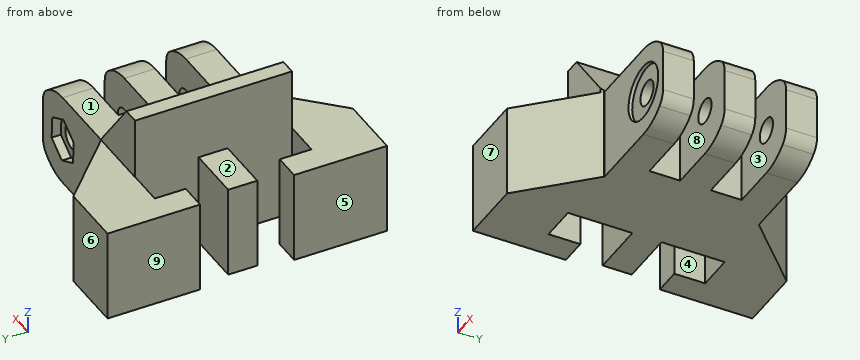
```python
from build123d import *

# Parameters (mm, degrees)
BOSS_EXTRUDE1_DEPTH = 15
FILLET1_R           = 7.5
SKETCH2_R           = 2
CUT_EXTRUDE1_DEPTH  = 56.055379886
SKETCH3_R           = 4.5
CUT_EXTRUDE2_DEPTH  = 0.6
CUT_EXTRUDE3_DEPTH  = 1.5
SKETCH5_W           = 11.340962939
SKETCH5_H           = 24.83561836
CUT_EXTRUDE4_DEPTH  = 56.308893581
FILLET2_R           = 3
SKETCH6_W           = 2.415249458
SKETCH6_H           = 25.484257417
BOSS_EXTRUDE2_DEPTH = 10
CHAMFER1_SIZE       = 8
CHAMFER1_SIZE_2     = 10.239533058


# Some blends are built 0.0001 mm under size
with BuildPart() as part:
    # Sketch1 → Boss-Extrude1 (new body)
    with BuildSketch(Plane.XY):
        Polygon((27.272753899, 35.386642786), (20.490738927, 35.386642786), (20.490738927, 35.487239574), (10.340798609, 45.376041655), (0, 45.376041655), (0, 30.338888881), (4.365624999, 30.338888881), (4.365624999, 35.365972213), (10.274652775, 35.365972213), (10.274652775, 25.091319438), (1.278819444, 25.091319438), (1.278819444, 20.372916662), (10.274652775, 20.372916662), (10.274652775, 9.921874998), (4.365624999, 9.921874998), (4.365624999, 15.081249996), (0, 15.081249996), (0, 0), (10.340798609, 0), (20.490738927, 10.304280596), (20.490738927, 10.386962888), (27.272753899, 10.386962888), (39.772593849, 10.386962888), (39.772593849, 15.38338487), (24.772648106, 15.38338487), (24.772648106, 20.383251948), (39.772593849, 20.383251948), (39.772593849, 22.886802837), (39.772593849, 25.362792962), (24.772648106, 25.362792962), (24.772648106, 30.36266004), (39.772593849, 30.36266004), (39.772593849, 35.386642786), align=None)
    extrude(amount=BOSS_EXTRUDE1_DEPTH)

    # Fillet1
    fillet1_edges = [part.edges().sort_by_distance(p)[0] for p in [
        (39.772593849, 32.874651413, 0),
        (39.772593849, 22.873022455, 0),
        (39.772593849, 12.885173879, 0),
        (39.772593849, 32.874651413, 15),
        (39.772593849, 22.873022455, 15),
        (39.772593849, 12.885173879, 15),
    ]]
    fillet(fillet1_edges, radius=FILLET1_R - 0.0001)  # a hair under: the kernel refuses the full size

    # Sketch2 → Cut-Extrude1 (cut, through all)
    with BuildSketch(Plane.XZ.offset(-10.386962888)):
        with Locations(Location((32.272593849, 7.5, 0), (0, 0, 270))):
            Circle(SKETCH2_R)
    extrude(amount=-CUT_EXTRUDE1_DEPTH, mode=Mode.SUBTRACT)

    # Sketch3 → Cut-Extrude2 (cut)
    with BuildSketch(Plane(origin=(0, 10.386962888, 0), x_dir=(-1, 0, 0), z_dir=(0, -1, 0))):
        with Locations(Location((-32.272593849, -7.5, 0), (0, 0, 90))):
            Circle(SKETCH3_R)
    extrude(amount=-CUT_EXTRUDE2_DEPTH, mode=Mode.SUBTRACT)

    # Sketch4 → Cut-Extrude3 (cut)
    with BuildSketch(Plane(origin=(0, 35.386642786, 0), x_dir=(1, 0, 0), z_dir=(0, 1, 0))):
        Polygon((35.624325063, -5.818215869), (32.491991675, -3.756423556), (29.14026046, -5.438207687), (28.920862634, -9.181784131), (32.053196023, -11.243576444), (35.404927237, -9.561792313), align=None)
    extrude(amount=-CUT_EXTRUDE3_DEPTH, mode=Mode.SUBTRACT)

    # Sketch5 → Cut-Extrude4 (cut, through all)
    with BuildSketch(Plane(origin=(0, 35.386642786, 0), x_dir=(1, 0, 0), z_dir=(0, 1, 0))):
        with Locations((43.904057381, -8.645001066)):
            Rectangle(SKETCH5_W, SKETCH5_H)
    extrude(amount=-CUT_EXTRUDE4_DEPTH, mode=Mode.SUBTRACT)

    # Fillet2
    fillet2_edges = [part.edges().sort_by_distance(p)[0] for p in [
        (38.233575911, 12.885173879, 2.948374426),
        (38.233575911, 12.885173879, 12.051625574),
        (38.233575911, 22.873022455, 12.051625574),
        (38.233575911, 22.873022455, 2.948374426),
        (38.233575911, 32.874651413, 12.051625574),
        (38.233575911, 32.874651413, 2.948374426),
    ]]
    fillet(fillet2_edges, radius=FILLET2_R)

    # Sketch6 → Boss-Extrude2 (add)
    with BuildSketch(Plane.XY.offset(15)):
        with Locations((11.482277504, 22.664003707)):
            Rectangle(SKETCH6_W, SKETCH6_H)
    extrude(amount=BOSS_EXTRUDE2_DEPTH)

    # Chamfer1
    # the kernel refuses this chamfer: 10.239533058, 8 mm, written as the material it adds along each edge
    with BuildSketch(Plane(origin=(12.689902233, 9.921874998, 15), x_dir=(0.9992360216896828, 0, -0.03908161918057676), z_dir=(0, 1, 0))) as chamfer1_piece_1_section:
        Polygon((CHAMFER1_SIZE * 0.99923602169, -CHAMFER1_SIZE * 0.0390816191806), (-CHAMFER1_SIZE_2 * 0.0390816191788, -CHAMFER1_SIZE_2 * 0.999236021645), (0, 0), align=None)
    chamfer1_piece_1 = extrude(amount=25.484257417, mode=Mode.PRIVATE)
    chamfer1_piece_1 = split(chamfer1_piece_1, bisect_by=Plane(origin=(20.793346788, 10.386962888, 14.678631533), z_dir=(0, 1, 0)), keep=Keep.TOP, mode=Mode.PRIVATE)
    chamfer1_piece_1 = split(chamfer1_piece_1, bisect_by=Plane(origin=(20.737221422, 10.554511111, 14.678631533), z_dir=(0.7124220763083485, -0.7017512274221556, 0)), keep=Keep.TOP, mode=Mode.PRIVATE)
    add(chamfer1_piece_1)
    with BuildSketch(Plane(origin=(12.689902233, 9.921874998, 15), x_dir=(0.9992360216896828, 0, -0.03908161918057676), z_dir=(0, 1, 0))) as chamfer1_piece_2_section:
        Polygon((CHAMFER1_SIZE * 0.99923602169, -CHAMFER1_SIZE * 0.0390816191806), (-CHAMFER1_SIZE_2 * 0.0390816191788, -CHAMFER1_SIZE_2 * 0.999236021645), (0, 0), align=None)
    chamfer1_piece_2 = extrude(amount=25.484257417, mode=Mode.PRIVATE)
    chamfer1_piece_2 = split(chamfer1_piece_2, bisect_by=Plane(origin=(15.274873459, 10.386962888, 18.392715242), z_dir=(0, -1, 0)), keep=Keep.TOP, mode=Mode.PRIVATE)
    chamfer1_piece_2 = split(chamfer1_piece_2, bisect_by=Plane(origin=(20.490738927, 10.154752313, 18.392715242), z_dir=(-1, 0, 0)), keep=Keep.TOP, mode=Mode.PRIVATE)
    chamfer1_piece_2 = split(chamfer1_piece_2, bisect_by=Plane(origin=(17.84740539, 7.620752455, 18.392715242), z_dir=(-0.7124220763083485, 0.7017512274221556, 0)), keep=Keep.TOP, mode=Mode.PRIVATE)
    chamfer1_piece_2 = split(chamfer1_piece_2, bisect_by=Plane(origin=(15.274873459, 10.154752313, 25), z_dir=(0, 0, -1)), keep=Keep.TOP, mode=Mode.PRIVATE)
    add(chamfer1_piece_2)
    with BuildSketch(Plane(origin=(12.689902233, 9.921874998, 15), x_dir=(0.9992360216896828, 0, -0.03908161918057676), z_dir=(0, 1, 0))) as chamfer1_piece_3_section:
        Polygon((CHAMFER1_SIZE * 0.99923602169, -CHAMFER1_SIZE * 0.0390816191806), (-CHAMFER1_SIZE_2 * 0.0390816191788, -CHAMFER1_SIZE_2 * 0.999236021645), (0, 0), align=None)
    chamfer1_piece_3 = extrude(amount=25.484257417, mode=Mode.PRIVATE)
    chamfer1_piece_3 = split(chamfer1_piece_3, bisect_by=Plane(origin=(20.673018583, 35.386642786, 14.762443719), z_dir=(0, -1, 0)), keep=Keep.TOP, mode=Mode.PRIVATE)
    chamfer1_piece_3 = split(chamfer1_piece_3, bisect_by=Plane(origin=(20.673018583, 10.386962888, 14.762443719), z_dir=(0, 1, 0)), keep=Keep.TOP, mode=Mode.PRIVATE)
    chamfer1_piece_3 = split(chamfer1_piece_3, bisect_by=Plane(origin=(20.490738927, 22.896544527, 14.762443719), z_dir=(1, 0, 0)), keep=Keep.TOP, mode=Mode.PRIVATE)
    chamfer1_piece_3 = split(chamfer1_piece_3, bisect_by=Plane(origin=(26.875918459, 16.786553348, 14.762443719), z_dir=(-0.7124220763083485, 0.7017512274221556, 0)), keep=Keep.TOP, mode=Mode.PRIVATE)
    chamfer1_piece_3 = split(chamfer1_piece_3, bisect_by=Plane(origin=(26.87746344, 29.264833071, 14.762443719), z_dir=(-0.6978327483962767, -0.7162607453055758, 0)), keep=Keep.TOP, mode=Mode.PRIVATE)
    add(chamfer1_piece_3)
    with BuildSketch(Plane(origin=(12.689902233, 9.921874998, 15), x_dir=(0.9992360216896828, 0, -0.03908161918057676), z_dir=(0, 1, 0))) as chamfer1_piece_4_section:
        Polygon((CHAMFER1_SIZE * 0.99923602169, -CHAMFER1_SIZE * 0.0390816191806), (-CHAMFER1_SIZE_2 * 0.0390816191788, -CHAMFER1_SIZE_2 * 0.999236021645), (0, 0), align=None)
    chamfer1_piece_4 = extrude(amount=25.484257417, mode=Mode.PRIVATE)
    chamfer1_piece_4 = split(chamfer1_piece_4, bisect_by=Plane(origin=(15.290163511, 35.386642786, 18.382453995), z_dir=(0, -1, 0)), keep=Keep.TOP, mode=Mode.PRIVATE)
    chamfer1_piece_4 = split(chamfer1_piece_4, bisect_by=Plane(origin=(15.290163511, 10.386962888, 18.382453995), z_dir=(0, 1, 0)), keep=Keep.TOP, mode=Mode.PRIVATE)
    chamfer1_piece_4 = split(chamfer1_piece_4, bisect_by=Plane(origin=(20.490738927, 22.886802837, 18.382453995), z_dir=(-1, 0, 0)), keep=Keep.TOP, mode=Mode.PRIVATE)
    chamfer1_piece_4 = split(chamfer1_piece_4, bisect_by=Plane(origin=(15.290163511, 22.886802837, 25), z_dir=(0, 0, -1)), keep=Keep.TOP, mode=Mode.PRIVATE)
    add(chamfer1_piece_4)
    with BuildSketch(Plane(origin=(12.689902233, 9.921874998, 15), x_dir=(0.9992360216896828, 0, -0.03908161918057676), z_dir=(0, 1, 0))) as chamfer1_piece_5_section:
        Polygon((CHAMFER1_SIZE * 0.99923602169, -CHAMFER1_SIZE * 0.0390816191806), (-CHAMFER1_SIZE_2 * 0.0390816191788, -CHAMFER1_SIZE_2 * 0.999236021645), (0, 0), align=None)
    chamfer1_piece_5 = extrude(amount=25.484257417, mode=Mode.PRIVATE)
    chamfer1_piece_5 = split(chamfer1_piece_5, bisect_by=Plane(origin=(20.802968311, 35.386642786, 14.671925701), z_dir=(0, -1, 0)), keep=Keep.TOP, mode=Mode.PRIVATE)
    chamfer1_piece_5 = split(chamfer1_piece_5, bisect_by=Plane(origin=(20.752085711, 35.232616736, 14.671925701), z_dir=(0.6978327483962767, 0.7162607453055758, 0)), keep=Keep.TOP, mode=Mode.PRIVATE)
    add(chamfer1_piece_5)
    with BuildSketch(Plane(origin=(12.689902233, 9.921874998, 15), x_dir=(0.9992360216896828, 0, -0.03908161918057676), z_dir=(0, 1, 0))) as chamfer1_piece_6_section:
        Polygon((CHAMFER1_SIZE * 0.99923602169, -CHAMFER1_SIZE * 0.0390816191806), (-CHAMFER1_SIZE_2 * 0.0390816191788, -CHAMFER1_SIZE_2 * 0.999236021645), (0, 0), align=None)
    chamfer1_piece_6 = extrude(amount=25.484257417, mode=Mode.PRIVATE)
    chamfer1_piece_6 = split(chamfer1_piece_6, bisect_by=Plane(origin=(15.290163511, 35.386642786, 18.382453995), z_dir=(0, 1, 0)), keep=Keep.TOP, mode=Mode.PRIVATE)
    chamfer1_piece_6 = split(chamfer1_piece_6, bisect_by=Plane(origin=(20.490738927, 35.396387601, 18.382453995), z_dir=(-1, 0, 0)), keep=Keep.TOP, mode=Mode.PRIVATE)
    chamfer1_piece_6 = split(chamfer1_piece_6, bisect_by=Plane(origin=(15.290163511, 35.396387601, 25), z_dir=(0, 0, -1)), keep=Keep.TOP, mode=Mode.PRIVATE)
    add(chamfer1_piece_6)


solid = part.part
```
Geometry check sheet. Reference: the model listing, model coordinates, mm. Face numbers are marked on the shaded views. A direction names the side the tool comes from. Coordinates: 2 decimals unless noted, no trailing zeros. Loops run counter-clockwise (first coordinate to the right, second up) from the corner with the lowest first, then second, coordinate; pieces in that order, holes last. Notation, with made-up numbers: (32.25, -11.5) - (37.25, -11.5) arc R22 ccw to (37.25, 26.5) - close; hole circle Ø6 at (72.5, 20.25). An arc over 180 degrees is marked (long way). One line per item, written item: value. Start each with the question number.
(1) Material ranges on line 1 (Y direction, x = 27, z = 14.5); line 2 (X direction, y = 10.85, z = 7.5); line 3 (Y direction, x = 4.5, z = 1.5), recorded low to high. Write a range as [from, to].
(2) Depth check by flat-ended pin: P1, Ø5, axis at x = 32.27, z = 7.5, coming from the +Y side; P2, Ø7, axis at x = 32.27, z = 7.5, coming from the -Y side; P3, Ø3, axis at y = 26.5, z = 8, coming from the -X side. Enter the tip coordinate at first touch or a pass-through.
(3) Cross-section at D-D on z = 7.5. Count the separate pieces of the cut face and the enclosed holes in it, plus the area to 3 significant figures.
(4) Cross-section at A-A on x = 3.5. Enter the section's corners in (y, z).
(5) Mould release check, pull along Y, two halves, no side actions. Record for the marked faces 6, 7, 8 and 9: released by +Y, released by -Y, zero draft, split by the parting line, or undercut.
(6) Cross-section at C-C on y = 29.5. Enter the section's corners in (x, z), plus the area to 3 significant figures.
(7) Tool access check on the marked faces 1, 2, 3, 4 and 5. Record the directions out of +Z, -Z, +X, -X, +Y, -Y that give a thin tool (end or side, any length) a straight path to the whole face; none if there is none.
(8) Cross-section at B-B on x = 9. Enter the section's corners in (y, z), plus the area to 3 significant figures.
Results below:
1. line 1: y = [10.39, 15.38], [20.38, 25.36], [30.36, 35.39]
1. line 2: x = [0, 4.37], [10.27, 27.77], [36.77, 38.23]
1. line 3: y = [0, 9.92], [20.37, 25.09], [35.37, 45.38]
2. P1: stops at y = 33.89
2. P2: stops at y = 10.99
2. P3: stops at x = 1.28
3. separate pieces: 4
3. enclosed holes: 0
3. area: 895 mm2
4. outline: (0, 0) - (15.08, 0) - (15.08, 15) - (0, 15) - close; (20.37, 0) - (25.09, 0) - (25.09, 15) - (20.37, 15) - close; (30.34, 0) - (45.38, 0) - (45.38, 15) - (30.34, 15) - close
5. face 6: released by +Y
5. face 7: released by -Y
5. face 8: undercut
5. face 9: zero draft
6. outline: (10.27, 0) - (24.77, 0) - (24.77, 15) - (20.69, 15) - (12.88, 25) - (10.27, 25) - close
6. area: 283 mm2
7. face 1: +Z, +X, +Y, -Y
7. face 2: +Z, -X, +Y, -Y
7. face 3: +Z, -Z, +X
7. face 4: +Z, -Z
7. face 5: +Z, -Z, -X, +Y, -Y
8. outline: (0, 0) - (9.92, 0) - (9.92, 15) - (0, 15) - close; (20.37, 0) - (25.09, 0) - (25.09, 15) - (20.37, 15) - close; (35.37, 0) - (45.38, 0) - (45.38, 15) - (35.37, 15) - close
8. area: 370 mm2
